```python
from build123d import *

# Parameters (mm, degrees)
ESQUISSE1_R        = 1.5
ESQUISSE1_R_2      = 0.75
BOSS_EXTRU_1_DEPTH = 2.54


with BuildPart() as part:
    # Esquisse1 → Boss.-Extru.1 (new body)
    with BuildSketch(Plane.XY):
        with BuildLine():
            Line((-3.5, 30), (-6.5, 0))
            ThreePointArc((-6.5, 0), (0, -6.5), (6.5, 0))
            Line((6.5, 0), (3.5, 30))
            ThreePointArc((3.5, 30), (0, 33.5), (-3.5, 30))
        make_face()
        Circle(ESQUISSE1_R, mode=Mode.SUBTRACT)
        with Locations((0, 13)):
            Circle(ESQUISSE1_R_2, mode=Mode.SUBTRACT)
        with Locations((0, 16)):
            Circle(ESQUISSE1_R_2, mode=Mode.SUBTRACT)
        with Locations((0, 19)):
            Circle(ESQUISSE1_R_2, mode=Mode.SUBTRACT)
        with Locations((0, 22)):
            Circle(ESQUISSE1_R_2, mode=Mode.SUBTRACT)
        with Locations((0, 25)):
            Circle(ESQUISSE1_R_2, mode=Mode.SUBTRACT)
        with Locations((0, 28)):
            Circle(ESQUISSE1_R_2, mode=Mode.SUBTRACT)
    extrude(amount=BOSS_EXTRU_1_DEPTH)


solid = part.part
```
Verification items for the finished model (mm, model axes). Coordinates: 2 decimals unless noted, no trailing zeros. Write each loop counter-clockwise with the first axis right and the second up, starting at its lowest first coordinate (ties: lowest second). Pieces come first, ordered by that corner, then holes. Notation, with made-up numbers: M 4,-29.5 L 14,-29.5 A28 cw 14,-0.5 Z; hole C -3,-13.75 d1. An arc over 180 degrees is marked long. One line per item, written item: value.
Item 1: Gauge pin test, flat end, axial feed: pin 1 Ø2 at (x, y) = (0, 25) entering from +Z. Record the tip position at first contact, or that the pin passes through.
Check sheet entries:
pin 1: stops at z = 2.54
Item 2: Section check B-B, the plane z = 0.5. Record the boundary of the cut face in (x, y).
Check sheet entries:
outline: M -6.5,0 A6.5 ccw 6.5,0 L 3.5,30 A3.5 ccw -3.5,30 Z; hole C 0,0 d3; hole C 0,13 d1.5; hole C 0,16 d1.5; hole C 0,19 d1.5; hole C 0,22 d1.5; hole C 0,25 d1.5; hole C 0,28 d1.5
Item 3: Mould release check, pull along Y, two halves, no side actions. Record for faces 1 (the cylindrical face through (-0.595, 27.544, 1.252)), 2 (the cylindrical face through (-0.1, -6.5, 1.3)), 3 (the flat face through (0, 14, 0)), 4 (the cylindrical face through (-0.163, 21.268, 1.252)): pulls with the +Y half, pulls with the -Y half, needs draft (parallel to the pull), parting line crosses it, or undercut.
Check sheet entries:
face 1: undercut
face 2: pulls with the -Y half
face 3: needs draft
face 4: undercut
Item 4: Scan lines: line 1 along X through (y, z) = (19.5, 2.15); line 2 along X through (y, z) = (11, 2.2); line 3 along Y through (x, z) = (2, 1.85). Record each from-to range of solid material in increasing order.
Check sheet entries:
line 1: x = -4.55 to -0.56, 0.56 to 4.55
line 2: x = -5.4 to 5.4
line 3: y = -6.18 to 32.87
Item 5: Section check A-A, the plane y = 16. Record the boundary of the cut face in (x, z), plus the area to 3 significant figures.
Check sheet entries:
outline: M -4.9,0 L -0.75,0 L -0.75,2.54 L -4.9,2.54 Z; M 0.75,0 L 4.9,0 L 4.9,2.54 L 0.75,2.54 Z
area: 21.1 mm^2
Item 6: Section check C-C, the plane x = 0. State how many separate pieces and enclosed holes the cut face has, plus the area to 3 significant figures.
Check sheet entries:
separate pieces: 8
enclosed holes: 0
area: 71.1 mm^2
Item 7: Section check D-D, the plane y = 28. Record the boundary of the cut face in (x, z), plus the area to 3 significant figures.
Check sheet entries:
outline: M -3.7,0 L -0.75,0 L -0.75,2.54 L -3.7,2.54 Z; M 0.75,0 L 3.7,0 L 3.7,2.54 L 0.75,2.54 Z
area: 15.0 mm^2
